Can you work these out from the model? Positions are in its coordinate system, mm. Face numbers are marked on the shaded views. A direction names the side the tool comes from. Coordinates: 2 decimals unless noted, no trailing zeros. Write each loop counter-clockwise with the first axis right and the second up, starting at its lowest first coordinate (ties: lowest second). Pieces come first, ordered by that corner, then holes. Notation, with made-up numbers: (42, -34.5) -> (101, -34.5) arc R22 ccw to (101, -23.5) -> close; hole circle Ø3 at (15.5, 51.25). An arc over 180 degrees is marked (long way). Answer as CSV lines item,"result". Start each with the question number.
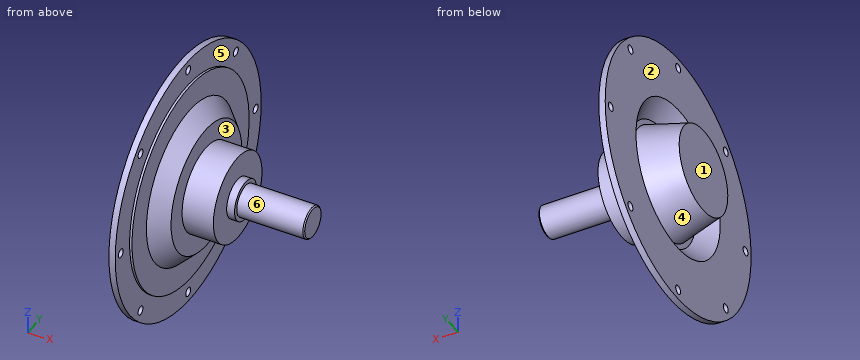
```python
from build123d import *

# Parameters (mm, degrees)
FASE1_SIZE                = 1.5
DURCHGANGSLOCH_F_R_M101_D = 11
KREISMUSTER1_COUNT        = 8


with BuildPart() as part:
    # Skizze3 → Rotation1 (revolve)
    with BuildSketch(Plane.XY, mode=Mode.PRIVATE) as rotation1_sk:
        Polygon((0, 132.5), (0, 165), (-8, 165), (-8, 95.443650814), (12, 75.443650814), (12, 68.933358006), (-40, 55), (-40, 0), (157.5, 0), (157.5, 20), (72.5, 20), (72.5, 25), (62.5, 25), (62.5, 55), (23, 55), (23, 80), (3, 100), (3, 132.5), align=None)
    revolve(rotation1_sk.sketch.rotate(Axis((-57.654973763, 0, 0), (1, 0, 0)), 90), axis=Axis((-57.654973763, 0, 0), (1, 0, 0)))

    # Fase1
    fase1_edges = [part.edges().sort_by_distance(p)[0] for p in [
        (157.5, 0, -20),
    ]]
    chamfer(fase1_edges, length=FASE1_SIZE)

    # Durchgangsloch für M101 (through all)
    with Locations(Plane(origin=(0, 0, 0), x_dir=(0, 0, -1), z_dir=(1, 0, 0))):
        with Locations((0, 152.5)):
            durchgangsloch_f_r_m101 = Hole(DURCHGANGSLOCH_F_R_M101_D / 2)

    # Kreismuster1: Durchgangsloch für M101 ×8 about axis
    kreismuster1_axis = Axis((0, 0, 0), (1, 0, 0))
    for i in range(1, KREISMUSTER1_COUNT):
        add(durchgangsloch_f_r_m101.rotate(kreismuster1_axis, i * 360 / KREISMUSTER1_COUNT), mode=Mode.SUBTRACT)


solid = part.part
```
Q1. Imagine slicing it at A-A (z = 152.5). Write out the boundary of the cut face in (x, y), then the cut area to 3 significant figures.
Q2. For pin 1 (17.5 mm diameter, centred on y = 152.5, z = 0, fed in from -X); pin 2 (2 mm diameter, centred on y = -87.5, z = 9, fed in from -X); pin 3 (10 mm diameter, centred on x = 103.5, z = 21.5, fed in from +Y), each with a flat end and sliding along its axis, tell me the tip position at first contact or that it passes through.
Q3. Which directions (+Z, -Z, +X, -X, +Y, -Y) give clear straight access to the entire face, cutting with the end or side of a thin tool? Please do the marked faces 1, 2 and 3.
Q4. I need wall thicknesses on L1, parallel to Y at x = -4, z = 0; L2, parallel to Y at x = 7.5, z = 62.5; L3, parallel to X at y = -101, z = 52. Which ranges of each line are inside material? Lowest first, please.
Q5. Imagine slicing it at C-C (y = 0). State how many separate pieces and enclosed holes the cut face has, then the cut area to 3 significant figures.
Q6. If we mould it in two halves opening along Z, with no side actions, what happens to the marked faces 4, 5 and 6? For each: released by +Z, released by -Z, zero draft, split by the parting line, or undercut.
Entries:
1,outline,"(-8, -63) -> (0, -63) -> (0, -5.5) -> (-8, -5.5) -> close; (-8, 5.5) -> (0, 5.5) -> (0, 63) -> (-8, 63) -> close"
1,area,"920 mm2"
2,pin 1,"x = -8"
2,pin 2,"x = -1.52"
2,pin 3,"y = 11.3"
3,face 1,"+Z, -Z, -X, +Y, -Y"
3,face 2,"-X"
3,face 3,"+X"
4,L1,"-165 to -158, -147 to -91.44, -64.65 to 64.65, 91.44 to 147, 158 to 165"
4,L2,"-72.21 to -49.85, -26.09 to 26.09, 49.85 to 72.21"
4,L3,"-8 to 3"
5,separate pieces,"3"
5,enclosed holes,"0"
5,area,"18,100 mm2"
6,face 4,"undercut"
6,face 5,"zero draft"
6,face 6,"split by the parting line"
